Source: CAD feature listing. Evaluate the final solid. Frame: model axes, mm. A direction names the side the tool comes from. Round coordinates to 2 decimals unless told otherwise and drop trailing zeros. Loops run counter-clockwise (first coordinate to the right, second up) from the corner with the lowest first, then second, coordinate; pieces in that order, holes last. Notation, with made-up numbers: (5.5, 63.25) - (41.5, 63.25) arc R25 ccw to (41.5, 77.25) - close; hole circle Ø11 at (-35.75, 71.25). An arc over 180 degrees is marked (long way). Use CSV: the item, a comma, the result in double quotes. Start each with the question number.
from build123d import *

# Parameters (mm, degrees)
SKETCH_4_R      = 9
EXTRUDE_3_DEPTH = 10
EXTRUDE_START   = 15
SKETCH_6_R      = 20
SKETCH_6_R_2    = 9
EXTRUDE_4_DEPTH = 15


with BuildPart() as part:
    # 草圖4 → 填料-伸長3 (new body)
    with BuildSketch(Plane.XY):
        with BuildLine():
            Line((2.498405104, 34.910714286), (3.655076706, 37.321447108))
            Line((3.655076706, 37.321447108), (5.153563847, 38.657997616))
            Line((5.153563847, 38.657997616), (7.044647753, 38.35847935))
            Line((7.044647753, 38.35847935), (8.056776892, 36.624286288))
            Line((8.056776892, 36.624286288), (8.411879546, 33.974111946))
            ThreePointArc((8.411879546, 33.974111946), (8.608704453, 32.11239943), (10.043052317, 30.90933678))
            ThreePointArc((10.043052317, 30.90933678), (11.910606599, 31.039546388), (13.164128454, 32.430012674))
            Line((13.164128454, 32.430012674), (15.00914593, 34.365324652))
            Line((15.00914593, 34.365324652), (16.84730871, 35.173401729))
            Line((16.84730871, 35.173401729), (18.553280148, 34.304165866))
            Line((18.553280148, 34.304165866), (18.979977034, 32.342085149))
            Line((18.979977034, 32.342085149), (18.498750817, 29.711886817))
            ThreePointArc((18.498750817, 29.711886817), (18.110641621, 27.880470756), (19.1030207, 26.293052317))
            ThreePointArc((19.1030207, 26.293052317), (20.91940735, 25.839783003), (22.541255192, 26.774835469))
            Line((22.541255192, 26.774835469), (24.894015376, 28.045284782))
            Line((24.894015376, 28.045284782), (26.891921615, 28.245788214))
            Line((26.891921615, 28.245788214), (28.245788214, 26.891921615))
            Line((28.245788214, 26.891921615), (28.045284782, 24.894015376))
            Line((28.045284782, 24.894015376), (26.774835469, 22.541255192))
            ThreePointArc((26.774835469, 22.541255192), (25.839783003, 20.91940735), (26.293052317, 19.1030207))
            ThreePointArc((26.293052317, 19.1030207), (27.880470756, 18.110641621), (29.711886817, 18.498750817))
            Line((29.711886817, 18.498750817), (32.342085149, 18.979977034))
            Line((32.342085149, 18.979977034), (34.304165866, 18.553280148))
            Line((34.304165866, 18.553280148), (35.173401729, 16.84730871))
            Line((35.173401729, 16.84730871), (34.365324652, 15.00914593))
            Line((34.365324652, 15.00914593), (32.430012674, 13.164128454))
            ThreePointArc((32.430012674, 13.164128454), (31.039546388, 11.910606599), (30.90933678, 10.043052317))
            ThreePointArc((30.90933678, 10.043052317), (32.11239943, 8.608704453), (33.974111946, 8.411879546))
            Line((33.974111946, 8.411879546), (36.624286288, 8.056776892))
            Line((36.624286288, 8.056776892), (38.35847935, 7.044647753))
            Line((38.35847935, 7.044647753), (38.657997616, 5.153563847))
            Line((38.657997616, 5.153563847), (37.321447108, 3.655076706))
            Line((37.321447108, 3.655076706), (34.910714286, 2.498405104))
            ThreePointArc((34.910714286, 2.498405104), (33.200942707, 1.735912687), (32.5, 0))
            ThreePointArc((32.5, 0), (33.200942707, -1.735912687), (34.910714286, -2.498405104))
            Line((34.910714286, -2.498405104), (37.321447108, -3.655076706))
            Line((37.321447108, -3.655076706), (38.657997616, -5.153563847))
            Line((38.657997616, -5.153563847), (38.35847935, -7.044647753))
            Line((38.35847935, -7.044647753), (36.624286288, -8.056776892))
            Line((36.624286288, -8.056776892), (33.974111946, -8.411879546))
            ThreePointArc((33.974111946, -8.411879546), (32.11239943, -8.608704453), (30.90933678, -10.043052317))
            ThreePointArc((30.90933678, -10.043052317), (31.039546388, -11.910606599), (32.430012674, -13.164128454))
            Line((32.430012674, -13.164128454), (34.365324652, -15.00914593))
            Line((34.365324652, -15.00914593), (35.173401729, -16.84730871))
            Line((35.173401729, -16.84730871), (34.304165866, -18.553280148))
            Line((34.304165866, -18.553280148), (32.342085149, -18.979977034))
            Line((32.342085149, -18.979977034), (29.711886817, -18.498750817))
            ThreePointArc((29.711886817, -18.498750817), (27.880470756, -18.110641621), (26.293052317, -19.1030207))
            ThreePointArc((26.293052317, -19.1030207), (25.839783003, -20.91940735), (26.774835469, -22.541255192))
            Line((26.774835469, -22.541255192), (28.045284782, -24.894015376))
            Line((28.045284782, -24.894015376), (28.245788214, -26.891921615))
            Line((28.245788214, -26.891921615), (26.891921615, -28.245788214))
            Line((26.891921615, -28.245788214), (24.894015376, -28.045284782))
            Line((24.894015376, -28.045284782), (22.541255192, -26.774835469))
            ThreePointArc((22.541255192, -26.774835469), (20.91940735, -25.839783003), (19.1030207, -26.293052317))
            ThreePointArc((19.1030207, -26.293052317), (18.110641621, -27.880470756), (18.498750817, -29.711886817))
            Line((18.498750817, -29.711886817), (18.979977034, -32.342085149))
            Line((18.979977034, -32.342085149), (18.553280148, -34.304165866))
            Line((18.553280148, -34.304165866), (16.84730871, -35.173401729))
            Line((16.84730871, -35.173401729), (15.00914593, -34.365324652))
            Line((15.00914593, -34.365324652), (13.164128454, -32.430012674))
            ThreePointArc((13.164128454, -32.430012674), (11.910606599, -31.039546388), (10.043052317, -30.90933678))
            ThreePointArc((10.043052317, -30.90933678), (8.608704453, -32.11239943), (8.411879546, -33.974111946))
            Line((8.411879546, -33.974111946), (8.056776892, -36.624286288))
            Line((8.056776892, -36.624286288), (7.044647753, -38.35847935))
            Line((7.044647753, -38.35847935), (5.153563847, -38.657997616))
            Line((5.153563847, -38.657997616), (3.655076706, -37.321447108))
            Line((3.655076706, -37.321447108), (2.498405104, -34.910714286))
            ThreePointArc((2.498405104, -34.910714286), (1.735912687, -33.200942707), (0, -32.5))
            ThreePointArc((0, -32.5), (-1.735912687, -33.200942707), (-2.498405104, -34.910714286))
            Line((-2.498405104, -34.910714286), (-3.655076706, -37.321447108))
            Line((-3.655076706, -37.321447108), (-5.153563847, -38.657997616))
            Line((-5.153563847, -38.657997616), (-7.044647753, -38.35847935))
            Line((-7.044647753, -38.35847935), (-8.056776892, -36.624286288))
            Line((-8.056776892, -36.624286288), (-8.411879546, -33.974111946))
            ThreePointArc((-8.411879546, -33.974111946), (-8.608704453, -32.11239943), (-10.043052317, -30.90933678))
            ThreePointArc((-10.043052317, -30.90933678), (-11.910606599, -31.039546388), (-13.164128454, -32.430012674))
            Line((-13.164128454, -32.430012674), (-15.00914593, -34.365324652))
            Line((-15.00914593, -34.365324652), (-16.84730871, -35.173401729))
            Line((-16.84730871, -35.173401729), (-18.553280148, -34.304165866))
            Line((-18.553280148, -34.304165866), (-18.979977034, -32.342085149))
            Line((-18.979977034, -32.342085149), (-18.498750817, -29.711886817))
            ThreePointArc((-18.498750817, -29.711886817), (-18.110641621, -27.880470756), (-19.1030207, -26.293052317))
            ThreePointArc((-19.1030207, -26.293052317), (-20.91940735, -25.839783003), (-22.541255192, -26.774835469))
            Line((-22.541255192, -26.774835469), (-24.894015376, -28.045284782))
            Line((-24.894015376, -28.045284782), (-26.891921615, -28.245788214))
            Line((-26.891921615, -28.245788214), (-28.245788214, -26.891921615))
            Line((-28.245788214, -26.891921615), (-28.045284782, -24.894015376))
            Line((-28.045284782, -24.894015376), (-26.774835469, -22.541255192))
            ThreePointArc((-26.774835469, -22.541255192), (-25.839783003, -20.91940735), (-26.293052317, -19.1030207))
            ThreePointArc((-26.293052317, -19.1030207), (-27.880470756, -18.110641621), (-29.711886817, -18.498750817))
            Line((-29.711886817, -18.498750817), (-32.342085149, -18.979977034))
            Line((-32.342085149, -18.979977034), (-34.304165866, -18.553280148))
            Line((-34.304165866, -18.553280148), (-35.173401729, -16.84730871))
            Line((-35.173401729, -16.84730871), (-34.365324652, -15.00914593))
            Line((-34.365324652, -15.00914593), (-32.430012674, -13.164128454))
            ThreePointArc((-32.430012674, -13.164128454), (-31.039546388, -11.910606599), (-30.90933678, -10.043052317))
            ThreePointArc((-30.90933678, -10.043052317), (-32.11239943, -8.608704453), (-33.974111946, -8.411879546))
            Line((-33.974111946, -8.411879546), (-36.624286288, -8.056776892))
            Line((-36.624286288, -8.056776892), (-38.35847935, -7.044647753))
            Line((-38.35847935, -7.044647753), (-38.657997616, -5.153563847))
            Line((-38.657997616, -5.153563847), (-37.321447108, -3.655076706))
            Line((-37.321447108, -3.655076706), (-34.910714286, -2.498405104))
            ThreePointArc((-34.910714286, -2.498405104), (-33.200942707, -1.735912687), (-32.5, 0))
            ThreePointArc((-32.5, 0), (-33.200942707, 1.735912687), (-34.910714286, 2.498405104))
            Line((-34.910714286, 2.498405104), (-37.321447108, 3.655076706))
            Line((-37.321447108, 3.655076706), (-38.657997616, 5.153563847))
            Line((-38.657997616, 5.153563847), (-38.35847935, 7.044647753))
            Line((-38.35847935, 7.044647753), (-36.624286288, 8.056776892))
            Line((-36.624286288, 8.056776892), (-33.974111946, 8.411879546))
            ThreePointArc((-33.974111946, 8.411879546), (-32.11239943, 8.608704453), (-30.90933678, 10.043052317))
            ThreePointArc((-30.90933678, 10.043052317), (-31.039546388, 11.910606599), (-32.430012674, 13.164128454))
            Line((-32.430012674, 13.164128454), (-34.365324652, 15.00914593))
            Line((-34.365324652, 15.00914593), (-35.173401729, 16.84730871))
            Line((-35.173401729, 16.84730871), (-34.304165866, 18.553280148))
            Line((-34.304165866, 18.553280148), (-32.342085149, 18.979977034))
            Line((-32.342085149, 18.979977034), (-29.711886817, 18.498750817))
            ThreePointArc((-29.711886817, 18.498750817), (-27.880470756, 18.110641621), (-26.293052317, 19.1030207))
            ThreePointArc((-26.293052317, 19.1030207), (-25.839783003, 20.91940735), (-26.774835469, 22.541255192))
            Line((-26.774835469, 22.541255192), (-28.045284782, 24.894015376))
            Line((-28.045284782, 24.894015376), (-28.245788214, 26.891921615))
            Line((-28.245788214, 26.891921615), (-26.891921615, 28.245788214))
            Line((-26.891921615, 28.245788214), (-24.894015376, 28.045284782))
            Line((-24.894015376, 28.045284782), (-22.541255192, 26.774835469))
            ThreePointArc((-22.541255192, 26.774835469), (-20.91940735, 25.839783003), (-19.1030207, 26.293052317))
            ThreePointArc((-19.1030207, 26.293052317), (-18.110641621, 27.880470756), (-18.498750817, 29.711886817))
            Line((-18.498750817, 29.711886817), (-18.979977034, 32.342085149))
            Line((-18.979977034, 32.342085149), (-18.553280148, 34.304165866))
            Line((-18.553280148, 34.304165866), (-16.84730871, 35.173401729))
            Line((-16.84730871, 35.173401729), (-15.00914593, 34.365324652))
            Line((-15.00914593, 34.365324652), (-13.164128454, 32.430012674))
            ThreePointArc((-13.164128454, 32.430012674), (-11.910606599, 31.039546388), (-10.043052317, 30.90933678))
            ThreePointArc((-10.043052317, 30.90933678), (-8.608704453, 32.11239943), (-8.411879546, 33.974111946))
            Line((-8.411879546, 33.974111946), (-8.056776892, 36.624286288))
            Line((-8.056776892, 36.624286288), (-7.044647753, 38.35847935))
            Line((-7.044647753, 38.35847935), (-5.153563847, 38.657997616))
            Line((-5.153563847, 38.657997616), (-3.655076706, 37.321447108))
            Line((-3.655076706, 37.321447108), (-2.498405104, 34.910714286))
            ThreePointArc((-2.498405104, 34.910714286), (-1.735912687, 33.200942707), (0, 32.5))
            ThreePointArc((0, 32.5), (1.735912687, 33.200942707), (2.498405104, 34.910714286))
        make_face()
        Circle(SKETCH_4_R, mode=Mode.SUBTRACT)
    extrude(amount=-EXTRUDE_3_DEPTH)

    # 草圖6 → 填料-伸長4 (add)
    with BuildSketch(Plane.XY.offset(EXTRUDE_START)):
        with Locations(Location((0, 0, 0), (0, 0, 180))):
            Circle(SKETCH_6_R)
        Circle(SKETCH_6_R_2, mode=Mode.SUBTRACT)
    extrude(amount=-EXTRUDE_4_DEPTH)


solid = part.part
1. Section query B-B on y = 21.5. Return the cut outline in (x, z).
2. Mould query, pull axis Y, two halves, no side actions, for faces 6 (the flat face through (-8.237, 35.281, -4.93)), 7 (the flat face through (27.4, 23.7, -4.9)), 8 (the flat face through (25.907, -28.147, -4.93)). Classes: +Y half, -Y half, draft (parallel to the pull), parting line (faces both ways), or undercut.
3. Reachability of faces 1 (the flat face through (-31.045, 18.743, -4.93)), 2 (the flat face through (28.144, -25.879, -4.93)), 3 (the flat face through (-34.764, 15.915, -4.93)), 4 (the flat face through (8.237, -35.281, -4.93)), 5 (the flat face through (-37.479, -7.558, -4.93)) from +Z, -Z, +X, -X, +Y, -Y: full face, straight path, thin tool, end or side. Return the list, or none.
4. Section query A-A on z = 4.5. Return the cut outline in (x, y).
5. Line query: line 1 along Y through (x, z) = (0, 1.75); line 2 along X through (y, z) = (3.5, 8.25); line 3 along X through (y, z) = (-4.5, 8.75). Output: solid intervals per line, ascending.
6. Contact query for flat-ended pins moving along their axis: P1, Ø5, axis at y = 22.5, z = -4.5, coming from the -X side; P2, Ø8, axis at x = 5.5, z = 5, coming from the -Y side; P3, Ø16, axis at x = 0, y = 0, coming from the -Z side. Output: stop coordinate, or through.
Values:
1,outline,"(-25.99, -10) - (25.99, -10) - (25.99, 0) - (-25.99, 0) - close"
2,face 6,"+Y half"
2,face 7,"undercut"
2,face 8,"-Y half"
3,face 1,"+Z, -Z, +Y"
3,face 2,"+Z, -Z, +X"
3,face 3,"+Z, -Z, -X"
3,face 4,"+Z, -Z, -Y"
3,face 5,"+Z, -Z, -X, -Y"
4,outline,"circle Ø40 at (0, 0); hole circle Ø18 at (0, 0)"
5,line 1,"y = -20 to -9, 9 to 20"
5,line 2,"x = -19.69 to -8.29, 8.29 to 19.69"
5,line 3,"x = -19.49 to -7.79, 7.79 to 19.49"
6,P1,"stops at x = -28.06"
6,P2,"stops at y = -19.94"
6,P3,"passes through"
